Autodesk Inventor part; units mm, degrees
ref_plane "YZ Plane" through (0, 0, 0) normal (1, 0, 0) x (0, 1, 0)
ref_plane "XZ Plane" through (0, 0, 0) normal (0, 1, 0) x (-1, 0, 0)
ref_plane "XY Plane" through (0, 0, 0) normal (0, 0, 1) x (1, 0, 0)
sketch "Sketch1" plane through (0, 0, 0) normal (0, 0, 1) x (1, 0, 0)
  line L0 (-38.9255, 12.5476) -> (38.9255, 12.5476)
  line L1 (38.9255, 12.5476) -> (38.9255, -12.5476)
  line L2 (38.9255, -12.5476) -> (-38.9255, -12.5476)
  line L3 (-38.9255, -12.5476) -> (-38.9255, 12.5476)
  point P0 (0, 0)
  point P1 (38.9255, 0)
  point P2 (0, 12.5476)
  dimension "d0" = 77.851
  dimension "d1" = 25.0952
extrude "Extrusion1" add sketch "Sketch1" against normal blind 5.334
sketch "Sketch2" plane through (0, 0, 0) normal (0, 0, 1) x (1, 0, 0)
  line L0 (-38.9255, 12.5476) -> (38.9255, 12.5476)
  line L1 (38.9255, -12.5476) -> (-38.9255, -12.5476)
  line L2 (-11.176, -6.1976) -> (11.176, -6.1976)
  line L3 (11.176, -6.1976) -> (11.176, -12.5476)
  line L4 (11.176, -12.5476) -> (-11.176, -12.5476)
  line L5 (-11.176, -12.5476) -> (-11.176, -6.1976)
  point P0 (0, 0)
  point P1 (0, -6.1976)
  point P2 (0, 12.5476)
  dimension "d4" = 22.352
  dimension "d5" = 6.35
extrude "Extrusion2" cut sketch "Sketch2" against normal blind 25.4
mirror "Mirror1" about plane through (0, 0, 0) normal (0, 1, 0) of "Extrusion2"
sketch "Sketch3" plane through (0, 0, 0) normal (0, 0, 1) x (1, 0, 0)
  line L0 (-54.4957, 0) -> (54.4957, 0)
  line L1 (0, 17.5666) -> (0, -17.5666)
  point P0 (0, 0)
  point P1 (-25.4, 0)
  dimension "d8" = 25.4
hole "Hole1" at (-25.4, 0, 0) direction (0, 0, -1) diameter 4.8006 end through all
mirror "Mirror2" about plane through (0, 0, 0) normal (1, 0, 0) of "Hole1"
chamfer "Chamfer1" distance 0.8128 angle 45 4 edges at (11.176, 12.5476, -2.667) (-11.176, 12.5476, -2.667) (11.176, -12.5476, -2.667) (-11.176, -12.5476, -2.667)
properties material "ACRYLIC, CLEAR"
Input: part model. Units: mm. Frame: model coordinates. A direction names the side the tool comes from. Give positions to 0.01 mm unless a question says otherwise; leave off trailing zeros. Order: outer loops, then holes, each group sorted by start corner. A loop starts at its lowest first (then second) coordinate and runs counter-clockwise, first axis right, second up. Notation, with made-up numbers: (74, 48) - (96, 48) arc R19 ccw to (96, 82) - close; hole circle Ø10 at (5.25, 78.5). An arc over 180 degrees is marked (long way). Put each result on its own line as item: value.
Item 1: Access query for faces 4 (the flat face through (-38.926, 0, -3)), 5 (the flat face through (0, 6.198, -3)), 6 (the flat face through (11.176, -9, -3)). Directions: +Z, -Z, +X, -X, +Y, -Y. A direction counts if a zero-diameter tool reaches every point of the face in a straight line with its end or side. Return the directions, or none.
Found:
face 4: +Z, -Z, -X, +Y, -Y
face 5: +Z, -Z, +Y
face 6: +Z, -Z, -Y
Item 2: Section query C-C, the plane z = -2.7. Return loops of the section in (x, y).
Found:
outline: (-38.93, -12.55) - (-11.99, -12.55) - (-11.18, -11.73) - (-11.18, -6.2) - (11.18, -6.2) - (11.18, -11.73) - (11.99, -12.55) - (38.93, -12.55) - (38.93, 12.55) - (11.99, 12.55) - (11.18, 11.73) - (11.18, 6.2) - (-11.18, 6.2) - (-11.18, 11.73) - (-11.99, 12.55) - (-38.93, 12.55) - close; hole circle Ø4.8 at (-25.4, 0); hole circle Ø4.8 at (25.4, 0)
Item 3: Contact query for flat-ended pins moving along their axis: pin 1 (1.6 mm diameter, centred on x = -3.5, z = -2.5, fed in from +Y); pin 2 (4 mm diameter, centred on x = -25.4, y = 0, fed in from -Z); pin 3 (1.6 mm diameter, centred on x = -4, z = -1.5, fed in from -Y). Output: stop coordinate, or through.
Found:
pin 1: stops at y = 6.2
pin 2: passes through
pin 3: stops at y = -6.2
Item 4: Section query B-B, the plane x = 25.4. Return loops of the section in (y, z), then the cut area to 3 significant figures.
Found:
outline: (-12.55, -5.33) - (-2.4, -5.33) - (-2.4, 0) - (-12.55, 0) - close; (2.4, -5.33) - (12.55, -5.33) - (12.55, 0) - (2.4, 0) - close
area: 108 mm^2
Item 5: Section query D-D, the plane y = 0. Return loops of the section in (x, z).
Found:
outline: (-38.93, -5.33) - (-27.8, -5.33) - (-27.8, 0) - (-38.93, 0) - close; (-23, -5.33) - (23, -5.33) - (23, 0) - (-23, 0) - close; (27.8, -5.33) - (38.93, -5.33) - (38.93, 0) - (27.8, 0) - close
Item 6: Draft query along X for faces 1 (the cylindrical face through (-23.27, -1.11, -2.7)), 2 (the flat face through (-26, 12.548, -3)), 3 (the flat face through (38.926, 0, -3)). Return one class per face: +X half, -X half, draft (parallel to the pull), parting line (faces both ways), or undercut.
Found:
face 1: undercut
face 2: draft
face 3: +X half
Item 7: Ray query, L1, parallel to X at y = 0, z = -4.75; L2, parallel to Y at x = -25.4, z = -3.6; L3, parallel to X at y = -1.25, z = -4.45. Return the intervals inside material, ascending. Write a range as from..to.
Found:
L1: x = -38.93..-27.8, -23..23, 27.8..38.93
L2: y = -12.55..-2.4, 2.4..12.55
L3: x = -38.93..-27.45, -23.35..23.35, 27.45..38.93
Item 8: Section query A-A, the plane y = -10.25. Return loops of the section in (x, z).
Found:
outline: (-38.93, -5.33) - (-11.18, -5.33) - (-11.18, 0) - (-38.93, 0) - close; (11.18, -5.33) - (38.93, -5.33) - (38.93, 0) - (11.18, 0) - close
